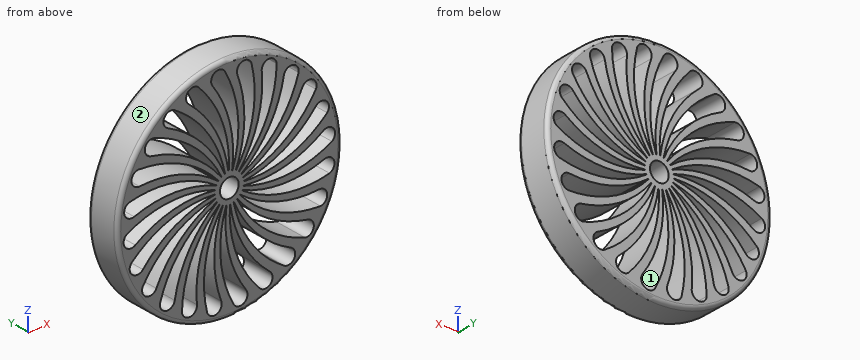
from build123d import *

# Parameters (mm, degrees)
SKETCH059_R        = 30
PAD036_DEPTH       = 9
POCKET022_DEPTH    = 100
POLARPATTERN_COUNT = 24
SKETCH061_R        = 2.5
POCKET023_DEPTH    = 100
FILLET_R           = 1


with BuildPart() as part:
    # Sketch059 → Pad036 (new body)
    with BuildSketch(Plane.XZ):
        Circle(SKETCH059_R)
    extrude(amount=PAD036_DEPTH)

    # Sketch060 → Pocket022 (cut)
    with BuildSketch(Plane.XZ):
        with BuildLine():
            ThreePointArc((0.256654, -3.915786), (3.732149, -14.491377), (10.824499, -23.071631))
            ThreePointArc((8.267765, -26.147848), (11.084241, -25.888106), (10.824499, -23.071631))
            ThreePointArc((0.15751, -3.928838), (1.873696, -15.89209), (8.267765, -26.147848))
            ThreePointArc((0.256654, -3.915786), (0.200556, -3.87274), (0.15751, -3.928838))
        make_face()
    pocket022 = extrude(amount=POCKET022_DEPTH, mode=Mode.SUBTRACT)

    # PolarPattern: Pocket022 ×24 about axis
    polarpattern_axis = Axis((0, 0, 0), (0, -1, 0))
    for i in range(1, POLARPATTERN_COUNT):
        add(pocket022.rotate(polarpattern_axis, i * 360 / POLARPATTERN_COUNT), mode=Mode.SUBTRACT)

    # Sketch061 → Pocket023 (cut)
    with BuildSketch(Plane.XZ):
        Circle(SKETCH061_R)
    extrude(amount=POCKET023_DEPTH, mode=Mode.SUBTRACT)

    # Fillet
    fillet_edges = [part.edges().sort_by_distance(p)[0] for p in [
        (-30, 0, 0),
        (-30, -9, 0),
    ]]
    fillet(fillet_edges, radius=FILLET_R)


with BuildPart() as part_1:
    # Body016 placement: moved
    add(part.part.moved(Location((-1, -101, 23))))


solid = part_1.part
The listing builds one solid part. Answer for the finished solid, in the listing's coordinates (mm). Face numbers are marked on the shaded views. Coordinates: 2 decimals unless noted, no trailing zeros. Use CSV: the item, a comma, the result in double quotes.
Q1. Section A-A (y = -104) is taken. Give the number of separate pieces and of enclosed holes in the cut face, then the cut area to 3 significant figures.
Here are the results:
separate pieces,"1"
enclosed holes,"25"
area,"1,430 mm2"
Q2. Given pin 1 Ø3 at (x, z) = (-1.5, 40.5) entering from +Y; pin 2 Ø2 at (y, z) = (-103.5, 31) entering from -X, each flat-ended and moving along its own axis, determine where each tip first touches the part or whether it passes through.
Here are the results:
pin 1,"y = -101"
pin 2,"x = -30.17"
Q3. Determine the mould class of the marked faces 1 and 2 for opening direction X: pulls with the +X half, pulls with the -X half, needs draft (parallel to the pull), parting line crosses it, or undercut.
Here are the results:
face 1,"undercut"
face 2,"parting line crosses it"
Q4. Straight lines are drawn through the part: L1, parallel to X at y = -103.5, z = 47; L2, parallel to X at y = -101.75, z = 0; L3, parallel to Z at x = 23, y = -102. For each, find the intervals that lie inside material, in ascending order.
Here are the results:
L1,"-19 to -12.45, -7.4 to -4.75, -0.62 to 1.64, 5.46 to 7.66, 11.63 to 17"
L2,"-20.21 to -13.59, -9.73 to -7.59, -3.93 to -1.75, 2.13 to 4.64, 9.74 to 13.56, 15.64 to 18.21"
L3,"5 to 10.37, 14.34 to 16.54, 20.36 to 22.62, 26.75 to 29.4, 34.45 to 41"
